For this review, take the finished solid that the model builds, in its own axes (mm). A direction names the side the tool comes from. Coordinates: 2 decimals unless noted, no trailing zeros. Write each loop counter-clockwise with the first axis right and the second up, starting at its lowest first coordinate (ties: lowest second). Pieces come first, ordered by that corner, then holes. Notation, with made-up numbers: (10.25, 47.5) -> (67.25, 47.5) arc R23 cw to (67.25, 64.5) -> close; hole circle Ø1 at (-13.5, 39). An arc over 180 degrees is marked (long way). Put each result on its own line as item: value. Start each with the question number.
Item 1: Consider section B-B on x = -41. Give the boundary of the cut face in (y, z), and give its area (3 significant figures).
Item 2: To check wall thickness, follow L1, parallel to X at y = -31, z = 6.25; L2, parallel to Y at x = 46.5, z = 16.25; L3, parallel to X at y = -37, z = 1.5. State the ranges of each line that lie inside material, in increasing order.
Item 3: The part is to be moulded in two halves that separate along Y. For faces 1 (the flat face through (-10, -35, 6)), 2 (the flat face through (0, -46, 2)), 3 (the flat face through (-2.751, -37.605, 3.085)), say which applies: +Y half, -Y half, draft (parallel to the pull), parting line (faces both ways), or undercut.
Item 4: Insertion check: P1, Ø4.5, axis at y = -34, z = 9, coming from the -X side; P2, Ø4.5, axis at y = -41, z = 6.5, coming from the +X side; P3, Ø2, axis at x = 16.5, z = 6, coming from the -Y side. Each pin has a flat end and moves straight along its axis. Give the tip position at first contact, or say it passes through.
Item 5: For faces 4 (the flat face through (-53, -13, 10)), 5 (the flat face through (-0.188, -32.221, 12.265)), 6 (the flat face through (52, -13, 10)), list the 3-axis set-ups (+Z, -Z, +X, -X, +Y, -Y) from which the entire face can be reached by the end or side of a thin tool; tool diameter is ignored.
Item 6: Consider section C-C on y = 0. Give the boundary of the cut face in (x, z).
Item 7: Consider section A-A on z = 10.25. Give the boundary of the cut face in (x, y), and give its area (3 significant figures).
```python
from build123d import *

# Parameters (mm, degrees)
CYLINDER_R               = 6
CYLINDER_DEPTH           = 15
CYLINDER_PLACEMENT_ANGLE = 29.9999898558
BOX_W                    = 30
BOX_H                    = 50
BOX_DEPTH                = 30
BOX_ROLL_ANGLE           = 29.9998791688
PAD_DEPTH                = 20
SKETCH001_R              = 3
POCKET_DEPTH             = 33.2329378555


with BuildPart() as cylinder:
    # Cylinder → Cylinder (new body)
    with BuildSketch(Plane.XY):
        Circle(CYLINDER_R)
    extrude(amount=CYLINDER_DEPTH)


with BuildPart() as cylinder_1:
    # Cylinder placement: moved
    add(cylinder.part.moved(Location((0, -32, -11))).rotate(Axis((0, -32, -11), (1, 0, 0)), CYLINDER_PLACEMENT_ANGLE))


with BuildPart() as box:
    # Box → Box (new body)
    with BuildSketch(Plane.XY):
        with Locations((15, 25)):
            Rectangle(BOX_W, BOX_H)
    extrude(amount=BOX_DEPTH)


with BuildPart() as box_1:
    # Box roll: moved
    add(box.part.rotate(Axis((0, 0, 0), (1, 0, 0)), BOX_ROLL_ANGLE))


with BuildPart() as box_2:
    # Box placement: moved
    add(box_1.part.moved(Location((-15, -50, 2))))


with BuildPart() as cut001:
    # Sketch → Pad (new body)
    with BuildSketch(Plane.XY):
        with BuildLine():
            Line((-79.5, 13), (79.5, 13))
            Line((79.5, 13), (79.5, 11.1))
            ThreePointArc((79.5, 11.1), (68.4, 0), (79.5, -11.1))
            Line((79.5, -13), (79.5, -11.1))
            Line((25.5184, -13), (79.5, -13))
            ThreePointArc((25.5184, -13), (14.5452341268, -17.5452341268), (10, -28.5184))
            Line((10, -46), (10, -28.5184))
            Line((-10, -46), (10, -46))
            Line((-10, -28.5184), (-10, -46))
            ThreePointArc((-10, -28.5184), (-14.5452341268, -17.5452341268), (-25.5184, -13))
            Line((-79.5, -13), (-25.5184, -13))
            Line((-79.5, -13), (-79.5, -11.1))
            ThreePointArc((-79.5, -11.1), (-68.4, 0), (-79.5, 11.1))
            Line((-79.5, 13), (-79.5, 11.1))
        make_face()
    extrude(amount=PAD_DEPTH)

    # Cut: cut Box
    add(box_2.part, mode=Mode.SUBTRACT)

    # Sketch001 → Pocket (cut, through all)
    with BuildSketch(Plane(origin=(0, -13.3659319768, 23.1505860246), x_dir=(1, 0, 0), z_dir=(0, -0.4999981736, 0.8660264582))):
        with Locations((0, -32.6825300346)):
            Circle(SKETCH001_R)
    extrude(amount=-POCKET_DEPTH, mode=Mode.SUBTRACT)

    # Cut001: cut Cylinder
    add(cylinder_1.part, mode=Mode.SUBTRACT)


solid = cut001.part
```
Return value:
1. outline: (-13, 0) -> (13, 0) -> (13, 20) -> (-13, 20) -> close
1. area: 520 mm^2
2. L1: -10 to 10
2. L2: -13 to 13
2. L3: -10 to -5.68, 5.68 to 10
3. face 1: draft
3. face 2: -Y half
3. face 3: undercut
4. P1: x = -10
4. P2: x = 10
4. P3: y = -16.67
5. face 4: +Z, -Z, -X, -Y
5. face 5: +Z, +X, -X, -Y
5. face 6: +Z, -Z, +X, -Y
6. outline: (-68.4, 0) -> (68.4, 0) -> (68.4, 20) -> (-68.4, 20) -> close
7. outline: (-79.5, -13) -> (-25.52, -13) arc R15.52 cw to (-10, -28.52) -> (-10, -35.71) -> (10, -35.71) -> (10, -28.52) arc R15.52 cw to (25.52, -13) -> (79.5, -13) -> (79.5, -11.1) arc R11.1 cw to (79.5, 11.1) -> (79.5, 13) -> (-79.5, 13) -> (-79.5, 11.1) arc R11.1 cw to (-79.5, -11.1) -> close
7. area: 4,300 mm^2
